Here's the drawing with two shaded views (mm, measured from the low corner). I have some questions. Round coordinates to 2 decimals unless told otherwise and drop trailing zeros. Order: outer loops, then holes, each group sorted by start corner. A loop starts at its lowest first (then second) coordinate and runs counter-clockwise, first axis right, second up.
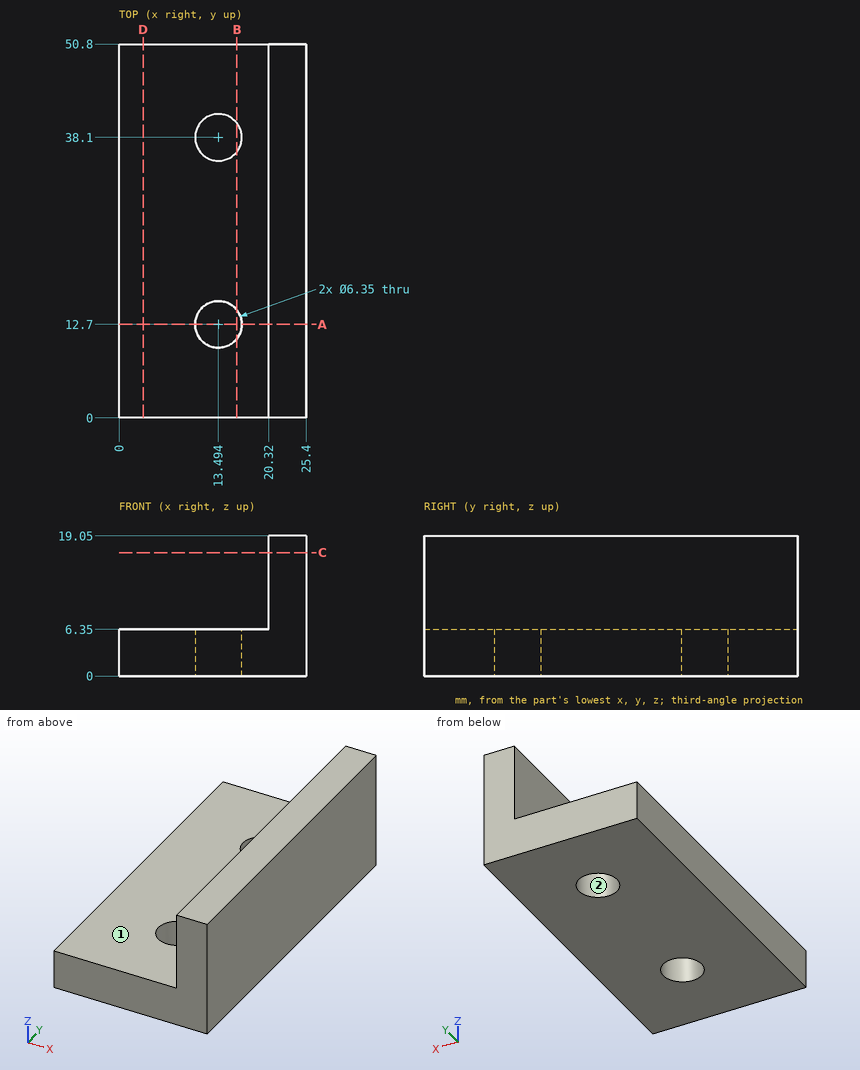
1. I'm going to push flat-ended pins straight in: P1, Ø7.5, axis at x = 13.49, y = 12.7, coming from the -Z side; P2, Ø6, axis at y = 36, z = 13.5, coming from the -X side; P3, Ø4, axis at x = 10, y = 41, coming from the +Z side. Where does each tip first touch, or does it pass through?
Evaluation:
P1: stops at z = 0
P2: stops at x = 20.32
P3: stops at z = 6.35
2. If we section it at A-A, the plane y = 12.7: Write out the boundary of the cut face in (x, z).
Evaluation:
outline: (0, 0) - (10.32, 0) - (10.32, 6.35) - (0, 6.35) - close; (16.67, 0) - (25.4, 0) - (25.4, 19.05) - (20.32, 19.05) - (20.32, 6.35) - (16.67, 6.35) - close
3. If we mould it in two halves opening along X, with no side actions, what happens to the marked faces 1 and 2? For each: released by +X, released by -X, zero draft, split by the parting line, or undercut.
Evaluation:
face 1: zero draft
face 2: undercut
4. I need wall thicknesses on probe 1 along Z at (x, y) = (4, 39.5); probe 2 along X at (y, z) = (12.7, 3); probe 3 along X at (y, z) = (46, 14.75). Which ranges of each line are inside material? Lowest first, please.
Evaluation:
probe 1: z = 0 to 6.35
probe 2: x = 0 to 10.32, 16.67 to 25.4
probe 3: x = 20.32 to 25.4
5. If we section it at D-D, the plane x = 3.25: Write out the boundary of the cut face in (y, z).
Evaluation:
outline: (0, 0) - (50.8, 0) - (50.8, 6.35) - (0, 6.35) - close
6. If we section it at C-C, the plane z = 16.75: Write out the boundary of the cut face in (x, y).
Evaluation:
outline: (20.32, 0) - (25.4, 0) - (25.4, 50.8) - (20.32, 50.8) - close
7. If we section it at B-B, the plane x = 16: Write out the boundary of the cut face in (y, z).
Evaluation:
outline: (0, 0) - (10.75, 0) - (10.75, 6.35) - (0, 6.35) - close; (14.65, 0) - (36.15, 0) - (36.15, 6.35) - (14.65, 6.35) - close; (40.05, 0) - (50.8, 0) - (50.8, 6.35) - (40.05, 6.35) - close
